Verification items for the finished model (mm, model axes). A direction names the side the tool comes from. Round coordinates to 2 decimals unless told otherwise and drop trailing zeros. Write each loop counter-clockwise with the first axis right and the second up, starting at its lowest first coordinate (ties: lowest second). Pieces come first, ordered by that corner, then holes. Notation, with made-up numbers: (77.5, 23) -> (133.5, 23) arc R10 ccw to (133.5, 28) -> close; hole circle Ø5 at (42, -3). An arc over 180 degrees is marked (long way). Answer as a JSON object with one key per item and string values. Group by question number.
(1) Sectioned sample at A-A on x = 0. Record the cut outline in (y, z), and give its area (3 significant figures).
(2) Sectioned sample at D-D on x = -8.5. Record the cut outline in (y, z).
(3) Gauge pin test, flat ends, axial feed: pin 1 Ø3.5 at (x, y) = (4, 31) entering from -Z; pin 2 Ø12.5 at (y, z) = (12, 24) entering from -X; pin 3 Ø1.1 at (x, y) = (2, -8) entering from +Z; pin 4 Ø10 at (x, z) = (-1.5, 24) entering from +Y. Record the tip position at first contact, or that the pin passes through.
(4) Sectioned sample at C-C on z = 17.5. Record the cut outline in (x, y).
(5) Set-up check for faces 1 (the face through (0, 33, 30)), 2 (the face through (0, 33, 33.5)), 3 (the face through (0, -14, 30)): record each of +Z, -Z, +X, -X, +Y, -Y from which the full face is reachable in a straight line by a thin tool's end or side.
(6) Sectioned sample at B-B on y = 0. Record the cut outline in (x, z), and give its area (3 significant figures).
(7) Scan lines: L1, parallel to X at y = 20, z = 16.5; L2, parallel to Z at x = -8.5, y = 0.5; L3, parallel to Z at x = 7, y = 32.5. Record each from-to range of solid material in increasing order. Write a range as from..to.
```python
from build123d import *

# Parameters (mm, degrees)
BOSS_EXTRUDE1_DEPTH = 19.999999553
SKETCH2_W           = 29.999999329
SKETCH2_H           = 7.099999115
CUT_EXTRUDE1_DEPTH  = 55.335457568
SKETCH3_W           = 7.599998266
SKETCH3_H           = 7.099999115
CUT_EXTRUDE2_DEPTH  = 55.335457568
SKETCH4_W           = 1.599997282
SKETCH4_H           = 3.620889969
CUT_EXTRUDE3_DEPTH  = 55.335457568
BOSS_EXTRUDE2_REACH = 56.335
SKETCH6_W           = 3.500001505
SKETCH6_H           = 7.10000284
SKETCH7_R           = 4
BOSS_EXTRUDE3_DEPTH = 7
MOVE_FACE2_BY       = 6
MOVE_FACE3_BY       = 6


with BuildPart() as part:
    # Sketch1 → Boss-Extrude1 (new body)
    with BuildSketch(Plane(origin=(10, 0, 0), x_dir=(0, 0, -1), z_dir=(1, 0, 0))):
        Polygon((0, 29.379108921), (-35.59999913, 29.379108921), (-41.0999991, 7.000000216), (-41.0999991, -17.7208893), (0, -17.7208893), align=None)
    extrude(amount=-BOSS_EXTRUDE1_DEPTH)

    # Sketch2 → Cut-Extrude1 (cut, through all)
    with BuildSketch(Plane(origin=(10, 0, 0), x_dir=(0, 0, -1), z_dir=(1, 0, 0))):
        with Locations((-14.999999665, -14.170889742)):
            Rectangle(SKETCH2_W, SKETCH2_H)
    extrude(amount=-CUT_EXTRUDE1_DEPTH, mode=Mode.SUBTRACT)

    # Sketch3 → Cut-Extrude2 (cut, through all)
    with BuildSketch(Plane(origin=(10, 0, 0), x_dir=(0, 0, -1), z_dir=(1, 0, 0))):
        with Locations((-37.299999967, -14.170889742)):
            Rectangle(SKETCH3_W, SKETCH3_H)
    extrude(amount=-CUT_EXTRUDE2_DEPTH, mode=Mode.SUBTRACT)

    # Sketch4 → Cut-Extrude3 (cut, through all)
    with BuildSketch(Plane(origin=(10, 0, 0), x_dir=(0, 0, -1), z_dir=(1, 0, 0))):
        with Locations((-40.300000459, -8.810445201)):
            Rectangle(SKETCH4_W, SKETCH4_H)
    extrude(amount=-CUT_EXTRUDE3_DEPTH, mode=Mode.SUBTRACT)

    # Boss-Extrude2: up to this plane
    boss_extrude2_end = Plane(origin=(-9.873244788, 0, -0.038787862), z_dir=(-0.9999922832070416, 0, -0.003928552706520363))
    # Sketch6 → Boss-Extrude2 (add, up to the surface)
    with BuildSketch(Plane(origin=(10, 0, 0), x_dir=(0, 0, -1), z_dir=(1, 0, 0)), mode=Mode.PRIVATE) as boss_extrude2_sk1:
        with Locations((-31.750000082, 32.929110341)):
            Rectangle(SKETCH6_W, SKETCH6_H)
    boss_extrude2_tool1 = split(extrude(boss_extrude2_sk1.sketch, amount=-BOSS_EXTRUDE2_REACH, mode=Mode.PRIVATE), bisect_by=boss_extrude2_end, keep=Keep.BOTH, mode=Mode.PRIVATE)
    add(boss_extrude2_tool1.solids().sort_by_distance((10, 32.92911, 31.75))[0])

    # Sketch7 → Boss-Extrude3 (add)
    with BuildSketch(Plane.XY.offset(41.0999991)):
        Circle(SKETCH7_R)
    extrude(amount=BOSS_EXTRUDE3_DEPTH)

    # Move Face2: a face moved outward by 6.0
    extrude(part.faces().sort_by_distance((0, 0, 48.0999991))[0], amount=MOVE_FACE2_BY, dir=(0, 0, 1))

    # Move Face3: a face moved inward by 6.0
    extrude(part.faces().sort_by_distance((0, 0, 54.0999991))[0], amount=MOVE_FACE3_BY, dir=(0, 0, -1), mode=Mode.SUBTRACT)


solid = part.part
```
Computed values:
{
 "1": {"outline": "(-17.72, 30) -> (-10.62, 30) -> (-10.62, 0) -> (29.38, 0) -> (29.38, 30) -> (36.48, 30) -> (36.48, 33.5) -> (29.38, 33.5) -> (29.38, 35.6) -> (7, 41.1) -> (4, 41.1) -> (4, 48.1) -> (-4, 48.1) -> (-4, 41.1) -> (-7, 41.1) -> (-7, 39.5) -> (-10.62, 39.5) -> (-10.62, 33.5) -> (-17.72, 33.5) -> close", "area": "1,680 mm2"},
 "2": {"outline": "(-17.72, 30) -> (-10.62, 30) -> (-10.62, 0) -> (29.38, 0) -> (29.38, 30) -> (36.48, 30) -> (36.48, 33.5) -> (29.38, 33.5) -> (29.38, 35.6) -> (7, 41.1) -> (-7, 41.1) -> (-7, 39.5) -> (-10.62, 39.5) -> (-10.62, 33.5) -> (-17.72, 33.5) -> close"},
 "3": {"pin 1": "z = 0", "pin 2": "x = -10", "pin 3": "z = 39.5", "pin 4": "y = 29.38"},
 "4": {"outline": "(-10, -10.62) -> (10, -10.62) -> (10, 29.38) -> (-10, 29.38) -> close"},
 "5": {"face 1": "-Z, +X, -X, +Y", "face 2": "+Z, +X, -X, +Y", "face 3": "-Z, +X, -X, -Y"},
 "6": {"outline": "(-10, 0) -> (10, 0) -> (10, 41.1) -> (4, 41.1) -> (4, 48.1) -> (-4, 48.1) -> (-4, 41.1) -> (-10, 41.1) -> close", "area": "878 mm2"},
 "7": {"L1": "-10..10", "L2": "0..41.1", "L3": "30..33.5"}
}
